Geometry: final body of the model. Coordinates: model frame, mm. A direction names the side the tool comes from. Coordinates: 2 decimals unless noted, no trailing zeros. Write each loop counter-clockwise with the first axis right and the second up, starting at its lowest first coordinate (ties: lowest second). Pieces come first, ordered by that corner, then holes. Notation, with made-up numbers: (-39.5, 43.5) -> (-6.5, 43.5) arc R25 cw to (-6.5, 63.5) -> close; hole circle Ø2 at (-21, 64.5). An arc over 180 degrees is marked (long way). Answer as a JSON object with one key per item and string values. Group by question number.
```python
from build123d import *

# Parameters (mm, degrees)
REVOLUCI_N1_ANGLE       = 180
REVOLUCI_N2_ANGLE       = 10
SALIENTE_EXTRUIR1_DEPTH = 6
CORTAR_EXTRUIR1_START   = -167.998723797
CROQUIS4_R              = 3
CORTAR_EXTRUIR1_DEPTH   = 173.998723797


with BuildPart() as part:
    # Croquis1 → Revoluci_n1 (revolve)
    with BuildSketch(Plane.XY):
        Polygon((0, 0), (0, 6.651019047), (39.028344285, 130.433112926), (40.935778186, 129.831701327), align=None)
    revolve(axis=Axis((0, 0, 0), (0, 1, 0)), revolution_arc=REVOLUCI_N1_ANGLE)

    # Croquis2 → Revoluci_n2 (revolve)
    with BuildSketch(Plane.XY):
        Polygon((40.935778186, 129.831701327), (40.935778186, 139.677786606), (41.935778186, 139.677786606), (41.935778186, 129.677786606), (39.483848741, 121.901259921), (38.53013179, 122.201965721), align=None)
    revoluci_n2 = revolve(axis=Axis((0, 0, 0), (0, 1, 0)), revolution_arc=REVOLUCI_N2_ANGLE)

    # Croquis3 → Saliente-Extruir1 (add)
    with BuildSketch(Plane.XY):
        Polygon((40.935778186, 139.677786606), (41.935778186, 139.677786606), (41.935778186, 129.677786606), (39.483848741, 121.901259921), (38.53013179, 122.201965721), (40.935778186, 129.831701327), align=None)
    saliente_extruir1 = extrude(amount=SALIENTE_EXTRUIR1_DEPTH)

    # Croquis4 → Cortar-Extruir1 (cut)
    with BuildSketch(Plane.ZY.offset(-40.935778186).offset(CORTAR_EXTRUIR1_START)):
        with Locations(Location((0, 134.754743966, 0), (0, 0, 90))):
            Circle(CROQUIS4_R)
    cortar_extruir1 = extrude(amount=CORTAR_EXTRUIR1_DEPTH, mode=Mode.SUBTRACT)

    # Simetr_a1: Revoluci_n2, Saliente-Extruir1, Cortar-Extruir1 across plane
    add(revoluci_n2.mirror(Plane(origin=(0, 0, 0), x_dir=(0, 0, 1), z_dir=(1, 0, 0))))
    add(saliente_extruir1.mirror(Plane(origin=(0, 0, 0), x_dir=(0, 0, 1), z_dir=(1, 0, 0))))
    add(cortar_extruir1.mirror(Plane(origin=(0, 0, 0), x_dir=(0, 0, 1), z_dir=(1, 0, 0))), mode=Mode.SUBTRACT)


solid = part.part
```
Item 1: Section B-B on y = 106. Output: boundary loops of the cut face in (x, z), then the cut area to 3 significant figures.
Item 2: Contact query for flat-ended pins moving along their axis: pin 1 (10 mm diameter, centred on x = 13, z = -36, fed in from +Y); pin 2 (6 mm diameter, centred on x = 18, y = 121.5, fed in from -Z); pin 3 (10 mm diameter, centred on x = 14, y = 40.5, fed in from -Z). Output: stop coordinate, or through.
Item 3: Set-up query: faces 5 (the flat face through (-40.5, 130.83, -7.14)), 6 (the flat face through (-41.936, 135, 4)), 7 (the flat face through (-39.716, 125.963, 2.958)). Return all of +Z, -Z, +X, -X, +Y, -Y with unobstructed straight access to the full face (end or side cutting, diameter ignored); none if empty.
Item 4: Mould query, pull axis Y, two halves, no side actions, for faces 1 (the conical face through (40.542, 125.735, -3.497)), 2 (the flat face through (-40.936, 135, 4)), 3 (the cylindrical face through (41.389, 132.544, -2.028)), 4 (the flat face through (39.716, 125.963, 2.958)). Classes: +Y half, -Y half, draft (parallel to the pull), parting line (faces both ways), or undercut.
Item 5: Section A-A on x = 0. Output: boundary loops of the cut face in (y, z), then the cut area to 3 significant figures.
Item 6: Ray query, L1, parallel to X at y = 108, z = -3; L2, parallel to X at y = 115.5, z = -12; L3, parallel to Z at x = 1.5, y = 96. Return the intervals inside material, ascending. Write a range as [from, to].
Answer sheet:
{
 "1": {"outline": "(-33.42, 0) arc R33.42 ccw to (33.42, 0) -> (31.32, 0) arc R31.32 cw to (-31.32, 0) -> close", "area": "213 mm^2"},
 "2": {"pin 1": "stops at y = 130.43", "pin 2": "stops at z = -35.61", "pin 3": "stops at z = -9.53"},
 "3": {"face 5": "-Z, -Y", "face 6": "+Z, -Z, -X, +Y, -Y", "face 7": "+Z, +Y"},
 "4": {"face 1": "-Y half", "face 2": "draft", "face 3": "undercut", "face 4": "+Y half"},
 "5": {"outline": "(0, 0) -> (129.83, -40.94) -> (130.43, -39.03) -> (6.65, 0) -> close", "area": "266 mm^2"},
 "6": {"L1": "x = [-33.92, -31.81], [31.81, 33.92]", "L2": "x = [-34.38, -32.15], [32.15, 34.38]", "L3": "z = [-30.23, -28.13]"}
}
